from build123d import *

# Parameters (mm, degrees)
F0_W     = 254
F0_H     = 50.8
F1_DEPTH = 1828.7999629974
F2_R     = 30.48
F3_DEPTH = 127


# Not quite as in the source:
# - a feature names something its author has since deleted; it is built from what else it names


with BuildPart() as f1:
    # F0 (on Right) → F1 (new body)
    with BuildSketch(Plane.YZ):
        with Locations((-10.6218170047, -93.1090038955)):
            Rectangle(F0_W, F0_H)
    extrude(amount=F1_DEPTH)

    # F2 (on Top) → F3 (cut)
    with BuildSketch(Plane.XY):
        with Locations((139.7, 59.2281829953)):
            Circle(F2_R)
        with Locations((254, 59.2281829953)):
            Circle(F2_R)
        with Locations((196.9066466086, -55.0718170047)):
            Circle(F2_R)
        with Locations((311.2066466086, -55.0718170047)):
            Circle(F2_R)
        with Locations((425.5066466086, -55.0718170047)):
            Circle(F2_R)
        with Locations((539.8066466086, -55.0718170047)):
            Circle(F2_R)
        with Locations((482.6, 59.2281829953)):
            Circle(F2_R)
        with Locations((594.391644001, 59.8655641079)):
            Circle(F2_R)
        with Locations((654.1066466086, -55.0718170047)):
            Circle(F2_R)
        with Locations((768.4066466086, -55.0718170047)):
            Circle(F2_R)
        with Locations((882.7066466086, -55.0718170047)):
            Circle(F2_R)
        with Locations((825.5, 59.2281829953)):
            Circle(F2_R)
        with Locations((940.1113390923, 59.2281829953)):
            Circle(F2_R)
        with Locations((997.0066466086, -55.0718170047)):
            Circle(F2_R)
        with Locations((1111.3066466086, -55.0718170047)):
            Circle(F2_R)
        with Locations((1054.1, 58.8000789285)):
            Circle(F2_R)
        with Locations((1225.6066466086, -55.0718170047)):
            Circle(F2_R)
        with Locations((1339.9066466086, -55.0718170047)):
            Circle(F2_R)
        with Locations((1282.7, 59.2281829953)):
            Circle(F2_R)
        with Locations((1397, 59.2281829953)):
            Circle(F2_R)
        with Locations((1454.2066466086, -55.0718170047)):
            Circle(F2_R)
        with Locations((1568.5066466086, -55.0718170047)):
            Circle(F2_R)
        with Locations((1625.6, 59.2281829953)):
            Circle(F2_R)
        with Locations((1682.8066466086, -55.0718170047)):
            Circle(F2_R)
        with Locations((1739.9, 56.6691346467)):
            Circle(F2_R)
    extrude(amount=-F3_DEPTH, mode=Mode.SUBTRACT)


solid = f1.part
Build history of the part. All positions in model axes, mm. Coordinates: 2 decimals unless noted, no trailing zeros. Order: outer loops, then holes, each group sorted by start corner. A loop starts at its lowest first (then second) coordinate and runs counter-clockwise, first axis right, second up. Notation, with made-up numbers: (-8.5, 75) - (23.5, 75) arc R11 cw to (23.5, 85) - close; hole circle Ø10 at (1.5, 26.5). An arc over 180 degrees is marked (long way). Write item = value, one per line. Start each with the question number.
1) Two-plate mould, pull along X, no slides. Class faces 1 (the face through (902, -12, -118.509)), 2 (the face through (1423.756, -53.732, -92.753)): pulls with the +X half, pulls with the -X half, needs draft (parallel to the pull), parting line crosses it, or undercut.
2) Wall check: line 1 along Y through (x, z) = (138, -77.5); line 2 along Y through (x, z) = (788.5, -107). Give the ranges that are in metal, low to high. Write a range as from..to.
3) Saw through at B-B on x = 1555.5. Write the cut outline in (y, z).
4) Saw through at A-A on x = 482.6. Write the cut outline in (y, z), then the cut area to 3 significant figures.
From the geometry:
q1.face_1 = needs draft
q1.face_2 = undercut
q2.line_1 = -137.62..28.8, 89.66..116.38
q2.line_2 = -137.62..-77.99, -32.15..116.38
q3.outline = (-137.62, -118.51) - (-82.64, -118.51) - (-82.64, -67.71) - (-137.62, -67.71) - close; (-27.51, -118.51) - (116.38, -118.51) - (116.38, -67.71) - (-27.51, -67.71) - close
q4.outline = (-137.62, -118.51) - (28.75, -118.51) - (28.75, -67.71) - (-137.62, -67.71) - close; (89.71, -118.51) - (116.38, -118.51) - (116.38, -67.71) - (89.71, -67.71) - close
q4.area = 9,810 mm^2
